```python
from build123d import *

# Parameters (mm, degrees)
SKETCH_2_OUTSIDE_W  = 22.99
SKETCH_2_OUTSIDE_H  = 22.99
CUT_EXTRUDE_1_DEPTH = 28.964168144
CHAMFER_1_SIZE      = 0.8


with BuildPart() as part:
    # Эскиз1 → Повернуть1 (revolve)
    with BuildSketch(Plane.XY, mode=Mode.PRIVATE) as revolve_1_sk:
        Polygon((-5.45, 0), (-5.45, 7.19), (0, 7.19), (0, 5.948974596), (0.6, 5.788205081), (0.6, 4), (20.6, 4), (20.6, 0), align=None)
    revolve(revolve_1_sk.sketch.rotate(Axis((-1000, 0, 0), (1, 0, 0)), 90), axis=Axis((-1000, 0, 0), (1, 0, 0)))

    # Эскиз2 outside → Вырез-Вытянуть1 (cut, through all)
    with BuildSketch(Plane.ZY.offset(5.45)):
        Rectangle(SKETCH_2_OUTSIDE_W, SKETCH_2_OUTSIDE_H)
        Polygon((0, -7.19), (6.226722653, -3.595), (6.226722653, 3.595), (0, 7.19), (-6.226722653, 3.595), (-6.226722653, -3.595), align=None, mode=Mode.SUBTRACT)
    extrude(amount=-CUT_EXTRUDE_1_DEPTH, mode=Mode.SUBTRACT)

    # Эскиз4 → Вырез-Повернуть1 (revolve, cut)
    with BuildSketch(Plane.XY, mode=Mode.PRIVATE) as cut_revolve_1_sk:
        Polygon((-5.45, 6.04675), (-5.03389103, 7.19), (-5.45, 7.19), align=None)
    revolve(cut_revolve_1_sk.sketch.rotate(Axis((-1000, 0, 0), (1, 0, 0)), 299.999999983), axis=Axis((-1000, 0, 0), (1, 0, 0)), mode=Mode.SUBTRACT)

    # Фаска1
    chamfer_1_edges = [part.edges().sort_by_distance(p)[0] for p in [
        (20.6, 0, -4),
    ]]
    chamfer(chamfer_1_edges, length=CHAMFER_1_SIZE)


solid = part.part
```
Geometry check sheet. Reference: the model listing, model coordinates, mm. A direction names the side the tool comes from. Coordinates: 2 decimals unless noted, no trailing zeros. Order: outer loops, then holes, each group sorted by start corner. A loop starts at its lowest first (then second) coordinate and runs counter-clockwise, first axis right, second up. Notation, with made-up numbers: M 0,76.25 L 35,76.25 A24 cw 35,103.25 Z; hole C 46.25,66 d7. An arc over 180 degrees is marked long. One line per question, with ' | ' between items. Start each with the question number.
Item 1: Cross-section at B-B on x = 11. Enter the section's corners in (y, z).
Item 2: Set-up check for faces 1 (the flat face through (-3, 0, -6.227)), 2 (the flat face through (0.6, -3.94, -1.37)): record each of +Z, -Z, +X, -X, +Y, -Y from which the full face is reachable in a straight line by a thin tool's end or side.
Item 3: Gauge pin test, flat ends, axial feed: pin 1 (6 mm diameter, centred on x = 9.5, z = 0.5, fed in from -Y); pin 2 (4 mm diameter, centred on x = 10.5, y = -0.5, fed in from -Z); pin 3 (1 mm diameter, centred on x = 5.5, z = -3, fed in from +Y). Record the tip position at first contact, or that the pin passes through.
Item 4: Material ranges on L1, parallel to X at y = 2.5, z = 2; L2, parallel to Y at x = 15.5, z = 0; L3, parallel to X at y = 2.75, z = 5, recorded low to high. Write a range as [from, to].
Item 5: Cross-section at A-A on y = 0. Enter the section's corners in (x, z), then the cut area to 3 significant figures.
Findings:
1) outline: C 0,0 d8
2) face 1: -Z, +X, -X, +Y, -Y | face 2: +X
3) pin 1: stops at y = -4 | pin 2: stops at z = -4 | pin 3: stops at y = 3.12
4) L1: x = [-5.45, 20.6] | L2: y = [-4, 4] | L3: x = [-5.45, 0.6]
5) outline: M -5.45,-6.05 L -5.38,-6.23 L 0,-6.23 L 0,-5.95 L 0.6,-5.79 L 0.6,-4 L 19.8,-4 L 20.6,-3.2 L 20.6,3.2 L 19.8,4 L 0.6,4 L 0.6,5.79 L 0,5.95 L 0,6.23 L -5.38,6.23 L -5.45,6.05 Z | area: 234 mm²
